from build123d import *

# Parameters (mm, degrees)
ESQUISSE1_W             = 17
ESQUISSE1_H             = 59
BOSS_EXTRU_1_DEPTH      = 2
ESQUISSE2_W             = 8.5
ESQUISSE2_H             = 59
BOSS_EXTRU_2_DEPTH      = 6
ENL_V_MAT_EXTRU_1_DEPTH = 6
ESQUISSE4_R             = 2.25
ENL_V_MAT_EXTRU_4_DEPTH = 22
ESQUISSE6_R             = 3.75
ENL_V_MAT_EXTRU_5_DEPTH = 6


with BuildPart() as part:
    # Esquisse1 → Boss.-Extru.1 (new body)
    with BuildSketch(Plane.XY):
        with Locations((8.5, -29.5)):
            Rectangle(ESQUISSE1_W, ESQUISSE1_H)
    extrude(amount=BOSS_EXTRU_1_DEPTH)

    # Esquisse2 → Boss.-Extru.2 (add)
    with BuildSketch(Plane.XY.offset(2)):
        with Locations((4.25, -29.5)):
            Rectangle(ESQUISSE2_W, ESQUISSE2_H)
    extrude(amount=BOSS_EXTRU_2_DEPTH)

    # Esquisse3 → Enlèv. mat.-Extru.1 (cut)
    with BuildSketch(Plane.XY.offset(8)):
        Polygon((5.519925502, -9), (5.519925502, -22), (5.519925502, -23), (7.019925502, -23), (7.019925502, -9), align=None)
        with BuildLine():
            Line((3.5, -23), (2, -23))
            ThreePointArc((2, -23), (2.408191843, -24.372032093), (3.5, -25.297800743))
            Line((3.5, -25.297800743), (3.5, -23))
        make_face()
        with BuildLine():
            Line((5.519925502, -23), (5.519925502, -25.297800743))
            ThreePointArc((5.519925502, -25.297800743), (6.611733659, -24.372032093), (7.019925502, -23))
            Line((7.019925502, -23), (5.519925502, -23))
        make_face()
        Polygon((5.519925502, -36), (5.519925502, -37), (5.519925502, -50), (7.019925502, -50), (7.019925502, -36), align=None)
        Polygon((2, -36), (2, -59), (3.5, -59), (3.5, -37), (3.5, -36), align=None)
        with BuildLine():
            Line((3.5, -33.702199257), (3.5, -36))
            Line((3.5, -36), (4.368453888, -36))
            ThreePointArc((4.368453888, -36), (4.509962751, -35.990037249), (4.651471614, -36))
            Line((4.651471614, -36), (5.519925502, -36))
            Line((5.519925502, -36), (5.519925502, -33.702199257))
            ThreePointArc((5.519925502, -33.702199257), (4.509962751, -33.490037249), (3.5, -33.702199257))
        make_face()
        with BuildLine():
            ThreePointArc((3.5, -33.702199257), (2.408191843, -34.627967907), (2, -36))
            Line((2, -36), (3.5, -36))
            Line((3.5, -36), (3.5, -33.702199257))
        make_face()
        with BuildLine():
            ThreePointArc((7.019925502, -36), (6.611733659, -34.627967907), (5.519925502, -33.702199257))
            Line((5.519925502, -33.702199257), (5.519925502, -36))
            Line((5.519925502, -36), (7.019925502, -36))
        make_face()
        with BuildLine():
            Line((4.368453888, -23), (3.5, -23))
            Line((3.5, -23), (3.5, -25.297800743))
            ThreePointArc((3.5, -25.297800743), (4.509962751, -25.509962751), (5.519925502, -25.297800743))
            Line((5.519925502, -25.297800743), (5.519925502, -23))
            Line((5.519925502, -23), (4.651471614, -23))
            ThreePointArc((4.651471614, -23), (4.509962751, -23.009962751), (4.368453888, -23))
        make_face()
        Polygon((2, 0), (2, -23), (3.5, -23), (3.5, -22), (3.5, 0), align=None)
        with BuildLine():
            Line((3.5, -22), (3.5, -23))
            Line((3.5, -23), (4.368453888, -23))
            ThreePointArc((4.368453888, -23), (3.747419821, -22.662233372), (3.5, -22))
        make_face()
        with BuildLine():
            Line((5.519925502, -23), (5.519925502, -22))
            ThreePointArc((5.519925502, -22), (5.272505681, -22.662233372), (4.651471614, -23))
            Line((4.651471614, -23), (5.519925502, -23))
        make_face()
        with BuildLine():
            Line((3.5, -36), (3.5, -37))
            ThreePointArc((3.5, -37), (3.747419821, -36.337766628), (4.368453888, -36))
            Line((4.368453888, -36), (3.5, -36))
        make_face()
        with BuildLine():
            ThreePointArc((4.651471614, -36), (5.272505681, -36.337766628), (5.519925502, -37))
            Line((5.519925502, -37), (5.519925502, -36))
            Line((5.519925502, -36), (4.651471614, -36))
        make_face()
    extrude(amount=-ENL_V_MAT_EXTRU_1_DEPTH, mode=Mode.SUBTRACT)

    # Esquisse4 → Enlèv. mat.-Extru.4 (cut)
    with BuildSketch(Plane.XY.offset(8)):
        with Locations((8.5, -29.5)):
            Circle(ESQUISSE4_R)
        with Locations((8.5, -54)):
            Circle(ESQUISSE4_R)
        with Locations((8.5, -5)):
            Circle(ESQUISSE4_R)
    extrude(amount=-ENL_V_MAT_EXTRU_4_DEPTH, mode=Mode.SUBTRACT)

    # Esquisse6 → Enlèv. mat.-Extru.5 (cut)
    with BuildSketch(Plane.XY.offset(8)):
        with Locations((8.5, -29.5)):
            Circle(ESQUISSE6_R)
        with Locations((8.5, -5)):
            Circle(ESQUISSE6_R)
        with Locations((8.5, -54)):
            Circle(ESQUISSE6_R)
    extrude(amount=-ENL_V_MAT_EXTRU_5_DEPTH, mode=Mode.SUBTRACT)


solid = part.part
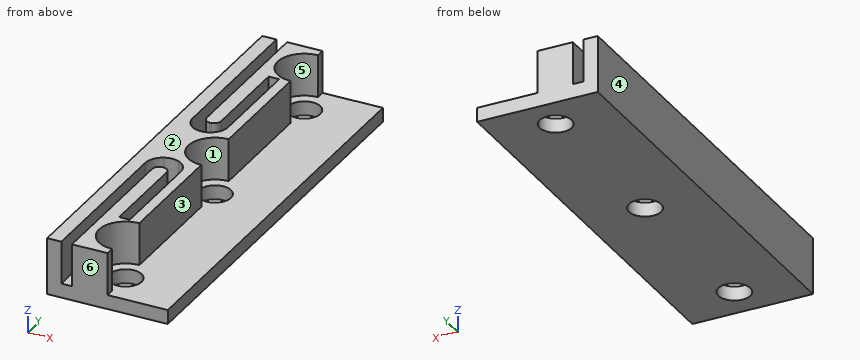
Read the model definition and answer for the solid it produces. Units are mm, in the model's axes. Face numbers are marked on the shaded views. A direction names the side the tool comes from. Coordinates: 2 decimals unless noted, no trailing zeros. Loops run counter-clockwise (first coordinate to the right, second up) from the corner with the lowest first, then second, coordinate; pieces in that order, holes last. Notation, with made-up numbers: (50, 42) -> (69, 42) arc R15 ccw to (69, 61) -> close; hole circle Ø5 at (-1, 69.25). An arc over 180 degrees is marked (long way). Write item = value, one per line. Start each with the question number.
1) The mould has two halves that part along Y. Classify the marked faces 4, 5 and 6: pulls with the +Y half, pulls with the -Y half, needs draft (parallel to the pull), parting line crosses it, or undercut.
2) The part is cut by section D-D, the plane y = -6. Determine the outline of the cut face in (x, z).
3) The part is cut by section B-B, the plane z = 0.75. Determine the outline of the cut face in (x, y).
4) For the marked faces 1, 2 and 3, determine the directions among +Z, -Z, +X, -X, +Y, -Y from which every point of the face is accessible in a straight line to the end or side of a thin tool.
5) The part is cut by section A-A, the plane y = -54. Determine the outline of the cut face in (x, z), plus the area to 3 significant figures.
6) The part is cut by section C-C, the plane x = 10. Determine the outline of the cut face in (y, z), plus the area to 3 significant figures.
7) Find the intervals of material crossed by L1, parallel to Y at x = 8.5, z = 1; L2, parallel to X at y = -21, z = 4.75; L3, parallel to Y at x = 4.5, z = 3.25, in increasing order. Write a range as from..to.
8) Given P1, Ø3, axis at x = 11, y = -25.5, coming from the -Z side; P2, Ø0.6, axis at y = -1, z = 5.5, coming from the +X side, each flat-ended and moving along its own axis, determine where each tip first touches the part or whether it passes through.
Result:
q1.face_4 = needs draft
q1.face_5 = undercut
q1.face_6 = pulls with the -Y half
q2.outline = (0, 0) -> (6.48, 0) -> (6.48, 2) -> (4.89, 2) -> (4.89, 8) -> (3.5, 8) -> (3.5, 2) -> (2, 2) -> (2, 8) -> (0, 8) -> close; (10.52, 0) -> (17, 0) -> (17, 2) -> (10.52, 2) -> close
q3.outline = (0, -59) -> (17, -59) -> (17, 0) -> (0, 0) -> close; hole circle Ø4.5 at (8.5, -54); hole circle Ø4.5 at (8.5, -29.5); hole circle Ø4.5 at (8.5, -5)
q4.face_1 = +Z, +X
q4.face_2 = +Z, +X, -X, +Y, -Y
q4.face_3 = +Z, +X, +Y, -Y
q5.outline = (0, 0) -> (6.25, 0) -> (6.25, 2) -> (4.75, 2) -> (4.75, 8) -> (3.5, 8) -> (3.5, 2) -> (2, 2) -> (2, 8) -> (0, 8) -> close; (10.75, 0) -> (17, 0) -> (17, 2) -> (10.75, 2) -> close
q5.area = 44.5 mm²
q6.outline = (-59, 0) -> (-55.68, 0) -> (-55.68, 2) -> (-59, 2) -> close; (-52.32, 0) -> (-31.18, 0) -> (-31.18, 2) -> (-52.32, 2) -> close; (-27.82, 0) -> (-6.68, 0) -> (-6.68, 2) -> (-27.82, 2) -> close; (-3.32, 0) -> (0, 0) -> (0, 2) -> (-3.32, 2) -> close
q6.area = 97.9 mm²
q7.L1 = -59..-56.25, -51.75..-31.75, -27.25..-7.25, -2.75..0
q7.L2 = 0..2, 3.5..5.52, 7.02..8.5
q7.L3 = -59..-35.99, -33.49..-25.51, -23.01..0
q8.P1 = 0
q8.P2 = 8.5
